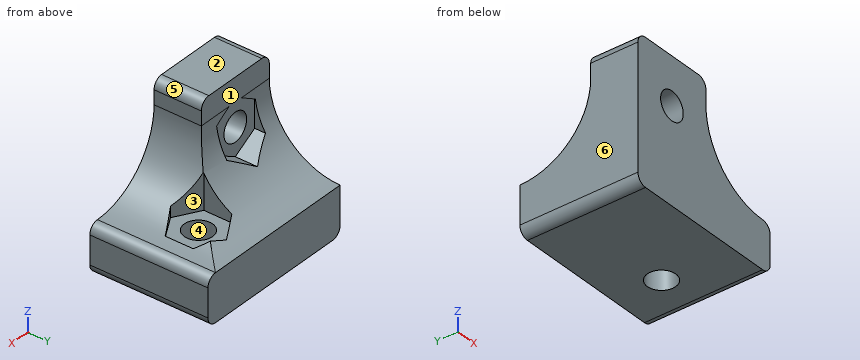
from build123d import *

# Parameters (mm, degrees)
SKETCH1_W           = 35
SKETCH1_H           = 25
BOSS_EXTRUDE1_DEPTH = 10
SKETCH2_R           = 3
CUT_EXTRUDE1_DEPTH  = 24.717082451
SKETCH3_W           = 18
SKETCH3_H           = 10
BOSS_EXTRUDE2_DEPTH = 20
SKETCH4_R           = 3
CUT_EXTRUDE2_DEPTH  = 38.831864876
FILLET2_R           = 15
FILLET3_R           = 2
CUT_EXTRUDE3_START  = -10
CUT_EXTRUDE3_DEPTH  = 27.912057753
CUT_EXTRUDE4_START  = -10
CUT_EXTRUDE4_DEPTH  = 33.793107057


# Some blends are built 0.0001 mm under size
with BuildPart() as part:
    # Sketch1 → Boss-Extrude1 (new body)
    with BuildSketch(Plane.XY):
        Rectangle(SKETCH1_W, SKETCH1_H)
    extrude(amount=BOSS_EXTRUDE1_DEPTH)

    # Sketch2 → Cut-Extrude1 (cut, through all)
    with BuildSketch(Plane.XY.offset(10)):
        with Locations((7.5, 2.5)):
            Circle(SKETCH2_R)
    extrude(amount=-CUT_EXTRUDE1_DEPTH, mode=Mode.SUBTRACT)

    # Sketch3 → Boss-Extrude2 (add)
    with BuildSketch(Plane.XY.offset(10)):
        with Locations((-8.5, -7.5)):
            Rectangle(SKETCH3_W, SKETCH3_H)
    extrude(amount=BOSS_EXTRUDE2_DEPTH)

    # Sketch4 → Cut-Extrude2 (cut, through all)
    with BuildSketch(Plane(origin=(0, -2.5, 0), x_dir=(1, 0, 0), z_dir=(0, 1, 0))):
        with Locations(Location((-8.5, -20, 0), (0, 0, 180))):
            Circle(SKETCH4_R)
    extrude(amount=-CUT_EXTRUDE2_DEPTH, mode=Mode.SUBTRACT)

    # Fillet2
    # the kernel refuses this fillet: 15 mm, written as the material it adds along each edge
    with BuildSketch(Plane(origin=(-17.5, -2.5, 10), x_dir=(0, 1, 0), z_dir=(1, 0, 0))) as fillet2_piece_1_section:
        with BuildLine():
            CenterArc((FILLET2_R, FILLET2_R), FILLET2_R, 180, 90)
            Line((0, FILLET2_R), (0, 0))
            Line((0, 0), (FILLET2_R, 0))
        make_face()
    fillet2_piece_1 = extrude(amount=18, mode=Mode.PRIVATE)
    fillet2_piece_1 = fillet2_piece_1 - Plane(origin=(-8.5, 1.000391612, 20), x_dir=(-1, 0, 0), z_dir=(0, 1, 0)) * Cylinder(3, 96, mode=Mode.PRIVATE)
    add(fillet2_piece_1)
    with BuildSketch(Plane(origin=(0.5, -2.5, 10), x_dir=(1, 0, 0), z_dir=(0, -1, 0))) as fillet2_piece_2:
        with BuildLine():
            CenterArc((FILLET2_R, FILLET2_R), FILLET2_R, 180, 90)
            Line((0, FILLET2_R), (0, 0))
            Line((0, 0), (FILLET2_R, 0))
        make_face()
    extrude(amount=10)
    with BuildSketch(Plane(origin=(-17.5, -2.5, 10), x_dir=(0, 1, 0), z_dir=(1, 0, 0))) as fillet2_piece_3a_section:
        with BuildLine():
            CenterArc((FILLET2_R, FILLET2_R), FILLET2_R, 180, 90)
            Line((0, FILLET2_R), (0, 0))
            Line((0, 0), (FILLET2_R, 0))
        make_face()
    fillet2_piece_3a = extrude(amount=55.5, mode=Mode.PRIVATE)
    fillet2_piece_3a = split(fillet2_piece_3a, bisect_by=Plane(origin=(17.5, 8.593163467, 10.419487564), z_dir=(-1, 0, 0)), keep=Keep.TOP, mode=Mode.PRIVATE)
    fillet2_piece_3a = fillet2_piece_3a - Plane(origin=(7.5, 2.5, 10.419487564), x_dir=(1, 0, 0), z_dir=(0, 0, 1)) * Cylinder(3, 171, mode=Mode.PRIVATE)
    fillet2_piece_3a = split(fillet2_piece_3a, bisect_by=Plane(origin=(0.5, 8.593163467, 10.419487564), z_dir=(1, 0, 0)), keep=Keep.TOP, mode=Mode.PRIVATE)
    with BuildSketch(Plane(origin=(0.5, 35, 10), x_dir=(1, 0, 0), z_dir=(0, -1, 0))) as fillet2_piece_3b_section:
        with BuildLine():
            CenterArc((FILLET2_R, FILLET2_R), FILLET2_R, 180, 90)
            Line((0, FILLET2_R), (0, 0))
            Line((0, 0), (FILLET2_R, 0))
        make_face()
    fillet2_piece_3b = extrude(amount=47.5, mode=Mode.PRIVATE)
    fillet2_piece_3b = split(fillet2_piece_3b, bisect_by=Plane(origin=(3.591954859, 12.5, 13.608813205), z_dir=(0, -1, 0)), keep=Keep.TOP, mode=Mode.PRIVATE)
    fillet2_piece_3b = fillet2_piece_3b - Plane(origin=(7.5, 2.5, 13.608813205), x_dir=(1, 0, 0), z_dir=(0, 0, 1)) * Cylinder(3, 155, mode=Mode.PRIVATE)
    fillet2_piece_3b = split(fillet2_piece_3b, bisect_by=Plane(origin=(3.591954859, -2.5, 13.608813205), z_dir=(0, 1, 0)), keep=Keep.TOP, mode=Mode.PRIVATE)
    fillet2_piece_3 = fillet2_piece_3a & fillet2_piece_3b
    add(fillet2_piece_3)

    # Fillet3
    fillet3_edges = [part.edges().sort_by_distance(p)[0] for p in [
        (17.5, 0, 0),
        (-17.5, 0, 0),
        (-17.5, -7.5, 30),
        (0.5, -7.5, 30),
        (17.5, 0, 10),
    ]]
    fillet(fillet3_edges, radius=FILLET3_R - 0.0001)  # a hair under: the kernel refuses the full size

    # Sketch5 → Cut-Extrude3 (cut, through all)
    with BuildSketch(Plane(origin=(0, 0, 0), x_dir=(-1, 0, 0), z_dir=(0, 0, -1)).offset(CUT_EXTRUDE3_START)):
        Polygon((-7.5, -3.417840259), (-2.375, -0.45892013), (-2.375, 5.45892013), (-7.5, 8.417840259), (-12.625, 5.45892013), (-12.625, -0.45892013), align=None)
    extrude(amount=-CUT_EXTRUDE3_DEPTH, mode=Mode.SUBTRACT)

    # Sketch6 → Cut-Extrude4 (cut, through all)
    with BuildSketch(Plane.XZ.offset(12.5).offset(CUT_EXTRUDE4_START)):
        Polygon((-8.5, 14.082159741), (-3.375, 17.04107987), (-3.375, 22.95892013), (-8.5, 25.917840259), (-13.625, 22.95892013), (-13.625, 17.04107987), align=None)
    extrude(amount=-CUT_EXTRUDE4_DEPTH, mode=Mode.SUBTRACT)


solid = part.part
Read the model definition and answer for the solid it produces. Units are mm, in the model's axes. Face numbers are marked on the shaded views. A direction names the side the tool comes from. Round coordinates to 2 decimals unless told otherwise and drop trailing zeros. Loops run counter-clockwise (first coordinate to the right, second up) from the corner with the lowest first, then second, coordinate; pieces in that order, holes last.
Q1. Each of these flat-tipped pins is pushed along its axis until it touches: pin 1 (5 mm diameter, centred on x = 1.5, y = -2.5, fed in from +Z); pin 2 (1.1 mm diameter, centred on y = -1.5, z = 20, fed in from +X); pin 3 (6 mm diameter, centred on y = 7.5, z = 16.5, fed in from -X); pin 4 (4 mm diameter, centred on x = 11, y = 1, fed in from +Z). Where does it stop, or does it pass through?
Q2. Section C-C on z = 2.75 is taken. Write down the section's boundary in (x, y), and give its area (3 significant figures).
Q3. Section B-B on x = -9.5 is taken. Write down the section's boundary in (y, z).
Q4. Determine the mould class of the marked faces 4, 5 and 6 for opening direction X: released by +X, released by -X, zero draft, split by the parting line, or undercut.
Q5. Consider probe 1 along X at (y, z) = (2.25, 5.5); probe 2 along Y at (x, z) = (7.5, 4.5); probe 3 along Z at (x, y) = (-8.5, -8.25). Determine where each line is inside the solid, lowest interval first.
Q6. Which of the six approach directions +Z, -Z, +X, -X, +Y, -Y give full straight-line access (tool end or side, diameter ignored) to the marked faces 1, 2 and 3?
Output:
1. pin 1: stops at z = 29.94
1. pin 2: stops at x = 1.56
1. pin 3: passes through
1. pin 4: stops at z = 10.28
2. outline: (-17.5, -12.5) - (17.5, -12.5) - (17.5, 12.5) - (-17.5, 12.5) - close; hole circle Ø6 at (7.5, 2.5)
2. area: 847 mm2
3. outline: (-12.5, 0) - (12.5, 0) - (12.5, 10) arc R15 cw to (1.63, 14.66) - (-2.5, 14.66) - (-2.5, 17.17) - (-12.5, 17.17) - close; (-12.5, 22.83) - (-2.5, 22.83) - (-2.5, 30) - (-12.5, 30) - close
4. face 4: undercut
4. face 5: released by +X
4. face 6: released by -X
5. probe 1: x = -17.5 to 4.51, 10.49 to 17.5
5. probe 2: y = -12.5 to -0.5, 5.5 to 12.5
5. probe 3: z = 0 to 17, 23 to 30
6. face 1: +Y
6. face 2: +Z, +X, -X, +Y, -Y
6. face 3: +Z
